The listing builds one solid part. Answer for the finished solid, in the listing's coordinates (mm). A direction names the side the tool comes from. Round coordinates to 2 decimals unless told otherwise and drop trailing zeros. Loops run counter-clockwise (first coordinate to the right, second up) from the corner with the lowest first, then second, coordinate; pieces in that order, holes last. Notation, with made-up numbers: (-9, -28.75) - (12, -28.75) arc R16 ccw to (12, -11.75) - close; hole circle Ø7 at (17.5, 8.25). An arc over 180 degrees is marked (long way). Write item = value, one per line. Start each with the question number.
1) For a pull along X with two mould halves and no side action, classify faces 1 (the cylindrical face through (-9.894, 10.502, -75.353)), 2 (the flat face through (1, 23, 49.932)), 3 (the flat face through (-26.19, 13.13, -24.66)) as released by +X, released by -X, zero draft, split by the parting line, or undercut.
2) Section C-C, the plane z = 0 is taken. Determine the outline of the cut face in (x, y), and give its area (3 significant figures).
3) Straight lines are drawn through the part: line 1 along Z through (x, y) = (0, 16); line 2 along X through (y, z) = (2, 0). For each, find the intervals that lie inside material, in ascending order.
4) Section B-B, the plane y = 14.5 is taken. Give the number of separate pieces and of enclosed holes in the cut face, and give its area (3 significant figures).
5) Section A-A, the plane x = 0 is taken. Determine the outline of the cut face in (y, z), and give its area (3 significant figures).
6) A tool of negligible diameter and unlimited length cuts with its end or side. For faces 4 (the flat face through (-1, 23, -49.932)), 5 (the flat face through (1, 7.5, 15)), 6 (the flat face through (-26, 13, 42.323)), from which of +Z, -Z, +X, -X, +Y, -Y can it reach the whole face along a straight path? Write none if from no direction.
7) Given pin 1 Ø1 at (y, z) = (4, 5.5) entering from -X; pin 2 Ø9 at (x, y) = (-35, 15.5) entering from +Z; pin 3 Ø1.5 at (y, z) = (9.5, 20) entering from +X, each flat-ended and moving along its own axis, determine where each tip first touches the part or whether it passes through.
8) Section D-D, the plane x = 27 is taken. Determine the outline of the cut face in (y, z), and give its area (3 significant figures).
from build123d import *

# Parameters (mm, degrees)
SKETCH1_R           = 76
BOSS_EXTRUDE1_DEPTH = 27.5
CUT_EXTRUDE4_DEPTH  = 8.89
SKETCH5_R           = 3
CUT_EXTRUDE5_DEPTH  = 20
CUT_EXTRUDE6_DEPTH  = 19.61
CUT_EXTRUDE7_DEPTH  = 19.61
SKETCH13_R          = 70
CUT_EXTRUDE9_DEPTH  = 7.5


with BuildPart() as part:
    # Sketch1 → Boss-Extrude1 (new body)
    with BuildSketch(Plane(origin=(0, 0, 0), x_dir=(1, 0, 0), z_dir=(0, 1, 0))):
        Circle(SKETCH1_R)
    extrude(amount=BOSS_EXTRUDE1_DEPTH)

    # Sketch2 → Cut-Extrude4 (cut)
    with BuildSketch(Plane(origin=(0, 27.5, 0), x_dir=(1, 0, 0), z_dir=(0, 1, 0))):
        with BuildLine():
            Line((-58.007955522, 49.931796385), (58.007955522, 49.931796385))
            ThreePointArc((58.007955522, 49.931796385), (107.939751907, 0), (58.007955522, -49.931796385))
            Line((58.007955522, -49.931796385), (-58.007955522, -49.931796385))
            ThreePointArc((-58.007955522, -49.931796385), (-107.939751907, 0), (-58.007955522, 49.931796385))
        make_face()
    extrude(amount=-CUT_EXTRUDE4_DEPTH, mode=Mode.SUBTRACT)

    # Sketch5 → Cut-Extrude5 (cut)
    with BuildSketch(Plane(origin=(0, 18.61, 0), x_dir=(1, 0, 0), z_dir=(0, 1, 0))):
        Circle(SKETCH5_R)
    extrude(amount=-CUT_EXTRUDE5_DEPTH, mode=Mode.SUBTRACT)

    # Sketch7 → Cut-Extrude6 (cut, through all)
    with BuildSketch(Plane(origin=(0, 18.61, 0), x_dir=(1, 0, 0), z_dir=(0, 1, 0))):
        Polygon((-50.125135648, 42.322849323), (-67.902913426, 6.490592664), (-22.902913426, 6.490592664), align=None)
        Polygon((67.902913426, 6.490592664), (22.902913426, 6.490592664), (50.125135648, 42.322849323), align=None)
        Polygon((50.125135648, -42.322849323), (67.902913426, -6.490592664), (22.902913426, -6.490592664), align=None)
        Polygon((-67.902913426, -6.490592664), (-22.902913426, -6.490592664), (-50.125135648, -42.322849323), align=None)
    extrude(amount=-CUT_EXTRUDE6_DEPTH, mode=Mode.SUBTRACT)

    # Sketch9 → Cut-Extrude7 (cut, through all)
    with BuildSketch(Plane(origin=(0, 18.61, 0), x_dir=(1, 0, 0), z_dir=(0, 1, 0))):
        Polygon((-12.5, 6.490592664), (-12.5, 42.322849323), (-39.5, 42.322849323), align=None)
        Polygon((12.5, 6.490592664), (39.5, 42.322849323), (12.5, 42.322849323), align=None)
        Polygon((12.5, -6.490592664), (12.5, -42.322849323), (39.5, -42.322849323), align=None)
        Polygon((-12.5, -6.490592664), (-39.5, -42.322849323), (-12.5, -42.322849323), align=None)
    extrude(amount=-CUT_EXTRUDE7_DEPTH, mode=Mode.SUBTRACT)

    # Sketch13 → Cut-Extrude9 (cut)
    with BuildSketch(Plane(origin=(0, 0, 0), x_dir=(-1, 0, 0), z_dir=(0, -1, 0))):
        Circle(SKETCH13_R)
    extrude(amount=-CUT_EXTRUDE9_DEPTH, mode=Mode.SUBTRACT)


solid = part.part
Geometry check:
q1.face_1 = split by the parting line
q1.face_2 = zero draft
q1.face_3 = undercut
q2.outline = (-76, 0) - (-70, 0) - (-70, 7.5) - (-3, 7.5) - (-3, 18.61) - (-76, 18.61) - close; (3, 7.5) - (70, 7.5) - (70, 0) - (76, 0) - (76, 18.61) - (3, 18.61) - close
q2.area = 1,710 mm2
q3.line_1 = -76 to -3, 3 to 76
q3.line_2 = -76 to -70, 70 to 76
q4.separate_pieces = 1
q4.enclosed_holes = 9
q4.area = 13,000 mm2
q5.outline = (0, -76) - (27.5, -76) - (27.5, -49.93) - (18.61, -49.93) - (18.61, -3) - (7.5, -3) - (7.5, -70) - (0, -70) - close; (0, 70) - (7.5, 70) - (7.5, 3) - (18.61, 3) - (18.61, 49.93) - (27.5, 49.93) - (27.5, 76) - (0, 76) - close
q5.area = 2,180 mm2
q6.face_4 = +X, -X, +Y
q6.face_5 = -Y
q6.face_6 = +Y, -Y
q7.pin_1 = -75.84
q7.pin_2 = 69.61
q7.pin_3 = 73.52
q8.outline = (0, -71.04) - (27.5, -71.04) - (27.5, -49.93) - (18.61, -49.93) - (18.61, -42.32) - (7.5, -42.32) - (7.5, -64.58) - (0, -64.58) - close; (0, 64.58) - (7.5, 64.58) - (7.5, 42.32) - (18.61, 42.32) - (18.61, 49.93) - (27.5, 49.93) - (27.5, 71.04) - (0, 71.04) - close; (7.5, -25.73) - (18.61, -25.73) - (18.61, -11.88) - (7.5, -11.88) - close; (7.5, -6.49) - (18.61, -6.49) - (18.61, 6.49) - (7.5, 6.49) - close; (7.5, 11.88) - (18.61, 11.88) - (18.61, 25.73) - (7.5, 25.73) - close
q8.area = 1,560 mm2
